```python
from build123d import *

# Parameters (mm, degrees)
F0_R     = 63.5
F1_DEPTH = 1.5875
F2_R     = 65.0875
F2_R_2   = 63.5
F3_DEPTH = 76.2


with BuildPart() as f1:
    # F0 (on Top) → F1 (new body)
    with BuildSketch(Plane.XY):
        with BuildLine():
            Line((152.4, 215.9), (152.4, 292.1))
            Line((152.4, 292.1), (88.9, 292.1))
            Line((88.9, 292.1), (88.9, 222.25))
            ThreePointArc((88.9, 222.25), (93.390128, 220.390128), (95.25, 215.9))
            Line((95.25, 215.9), (152.4, 215.9))
        make_face()
        with BuildLine():
            Line((88.9, 222.25), (88.9, 292.1))
            Line((88.9, 292.1), (-88.9, 292.1))
            Line((-88.9, 292.1), (-88.9, 222.25))
            ThreePointArc((-88.9, 222.25), (-84.409872, 220.390128), (-82.55, 215.9))
            ThreePointArc((-82.55, 215.9), (-84.409872, 211.409872), (-88.9, 209.55))
            Line((-88.9, 209.55), (-88.9, 6.35))
            ThreePointArc((-88.9, 6.35), (-84.409872, 4.490128), (-82.55, 0))
            ThreePointArc((-82.55, 0), (-84.409872, -4.490128), (-88.9, -6.35))
            Line((-88.9, -6.35), (-88.9, -184.15))
            ThreePointArc((-88.9, -184.15), (-84.409872, -186.009872), (-82.55, -190.5))
            Line((-82.55, -190.5), (82.55, -190.5))
            ThreePointArc((82.55, -190.5), (84.409872, -186.009872), (88.9, -184.15))
            Line((88.9, -184.15), (88.9, -6.35))
            ThreePointArc((88.9, -6.35), (82.55, 0), (88.9, 6.35))
            Line((88.9, 6.35), (88.9, 209.55))
            ThreePointArc((88.9, 209.55), (84.409872, 211.409872), (82.55, 215.9))
            ThreePointArc((82.55, 215.9), (84.409872, 220.390128), (88.9, 222.25))
        make_face()
        Circle(F0_R, mode=Mode.SUBTRACT)
        with BuildLine():
            Line((152.4, -152.4), (152.4, 215.9))
            Line((152.4, 215.9), (95.25, 215.9))
            ThreePointArc((95.25, 215.9), (93.390128, 211.409872), (88.9, 209.55))
            Line((88.9, 209.55), (88.9, 6.35))
            ThreePointArc((88.9, 6.35), (93.390128, 4.490128), (95.25, 0))
            ThreePointArc((95.25, 0), (93.390128, -4.490128), (88.9, -6.35))
            Line((88.9, -6.35), (88.9, -184.15))
            ThreePointArc((88.9, -184.15), (93.390128, -186.009872), (95.25, -190.5))
            Line((95.25, -190.5), (152.4, -190.5))
            Line((152.4, -190.5), (152.4, -152.4))
        make_face()
        with BuildLine():
            Line((-88.9, 222.25), (-88.9, 292.1))
            Line((-88.9, 292.1), (-152.4, 292.1))
            Line((-152.4, 292.1), (-152.4, 215.9))
            Line((-152.4, 215.9), (-95.25, 215.9))
            ThreePointArc((-95.25, 215.9), (-93.390128, 220.390128), (-88.9, 222.25))
        make_face()
        with BuildLine():
            Line((152.4, -292.1), (152.4, -190.5))
            Line((152.4, -190.5), (95.25, -190.5))
            ThreePointArc((95.25, -190.5), (93.390128, -194.990128), (88.9, -196.85))
            Line((88.9, -196.85), (88.9, -292.1))
            Line((88.9, -292.1), (152.4, -292.1))
        make_face()
        with BuildLine():
            Line((-95.25, 215.9), (-152.4, 215.9))
            Line((-152.4, 215.9), (-152.4, -152.4))
            Line((-152.4, -152.4), (-114.3, -190.5))
            Line((-114.3, -190.5), (-95.25, -190.5))
            ThreePointArc((-95.25, -190.5), (-93.390128, -186.009872), (-88.9, -184.15))
            Line((-88.9, -184.15), (-88.9, -6.35))
            ThreePointArc((-88.9, -6.35), (-95.25, 0), (-88.9, 6.35))
            Line((-88.9, 6.35), (-88.9, 209.55))
            ThreePointArc((-88.9, 209.55), (-93.390128, 211.409872), (-95.25, 215.9))
        make_face()
        with BuildLine():
            Line((12.7, -292.1), (88.9, -292.1))
            Line((88.9, -292.1), (88.9, -196.85))
            ThreePointArc((88.9, -196.85), (84.409872, -194.990128), (82.55, -190.5))
            Line((82.55, -190.5), (-82.55, -190.5))
            ThreePointArc((-82.55, -190.5), (-84.409872, -194.990128), (-88.9, -196.85))
            Line((-88.9, -196.85), (-88.9, -215.9))
            Line((-88.9, -215.9), (-12.7, -292.1))
            Line((-12.7, -292.1), (12.7, -292.1))
        make_face()
        with BuildLine():
            Line((-95.25, -190.5), (-114.3, -190.5))
            Line((-114.3, -190.5), (-88.9, -215.9))
            Line((-88.9, -215.9), (-88.9, -196.85))
            ThreePointArc((-88.9, -196.85), (-93.390128, -194.990128), (-95.25, -190.5))
        make_face()
    extrude(amount=F1_DEPTH)

    # F2 (on face) → F3 (join)
    with BuildSketch(Plane(origin=(0, 0, 0), x_dir=(1, 0, 0), z_dir=(0, 0, -1))):
        Circle(F2_R)
        Circle(F2_R_2, mode=Mode.SUBTRACT)
    extrude(amount=F3_DEPTH)


solid = f1.part
```
Can you work these out from the model? Positions are in its coordinate system, mm. Coordinates: 2 decimals unless noted, no trailing zeros. Loops run counter-clockwise (first coordinate to the right, second up) from the corner with the lowest first, then second, coordinate; pieces in that order, holes last.
Item 1: If we mould it in two halves opening along Y, with no side actions, what happens to faces 1 (the face through (-83.5, -221.3, 0.8)), 2 (the face through (-2, 69, 1.588)), 3 (the face through (-13.77, 61.99, -36.76)), 4 (the face through (-51.651, 39.605, -37.567))? For each: released by +Y, released by -Y, zero draft, split by the parting line, or undercut.
Answers below:
face 1: released by -Y
face 2: zero draft
face 3: undercut
face 4: split by the parting line
Item 2: Suppose I cut it at C-C (y = -98.5). Please give me the cut outline in (x, z), then the cut area to 3 significant figures.
Answers below:
outline: (-152.4, 0) - (152.4, 0) - (152.4, 1.59) - (-152.4, 1.59) - close
area: 484 mm2
Item 3: Suppose I cut it at B-B (z = -14). Please give me the cut outline in (x, y) (1 decimal).
Answers below:
outline: circle Ø130.2 at (0, 0); hole circle Ø127 at (0, 0)
Item 4: I'm going to push flat-ended pins straight in: pin 1 (10 mm diameter, centred on x = -21, y = -217, fed in from -Z); pin 2 (1.5 mm diameter, centred on y = -48.5, z = -67, fed in from -X). Where does each tip first touch, or does it pass through?
Answers below:
pin 1: stops at z = 0
pin 2: stops at x = -44.23
Item 5: Please list where these lines run through material, in increasing order: L1, parallel to Y at x = 0, z = -36; L2, parallel to Y at x = -4, z = -12.5.
Answers below:
L1: y = -65.09 to -63.5, 63.5 to 65.09
L2: y = -64.96 to -63.37, 63.37 to 64.96
Item 6: Suppose I cut it at D-D (x = -73). Please give me the cut outline in (y, z).
Answers below:
outline: (-231.8, 0) - (292.1, 0) - (292.1, 1.59) - (-231.8, 1.59) - close
Item 7: Suppose I cut it at A-A (x = 0). Please give me the cut outline in (y, z), then the cut area to 3 significant figures.
Answers below:
outline: (-292.1, 0) - (-65.09, 0) - (-65.09, -76.2) - (-63.5, -76.2) - (-63.5, 1.59) - (-292.1, 1.59) - close; (63.5, -76.2) - (65.09, -76.2) - (65.09, 0) - (292.1, 0) - (292.1, 1.59) - (63.5, 1.59) - close
area: 968 mm2
